Job drawing, mm, ordinate dimensions from the low corner. One solid piece. A direction names the side the tool comes from. Coordinates: 2 decimals unless noted, no trailing zeros. Write each loop counter-clockwise with the first axis right and the second up, starting at its lowest first coordinate (ties: lowest second). Pieces come first, ordered by that corner, then holes.
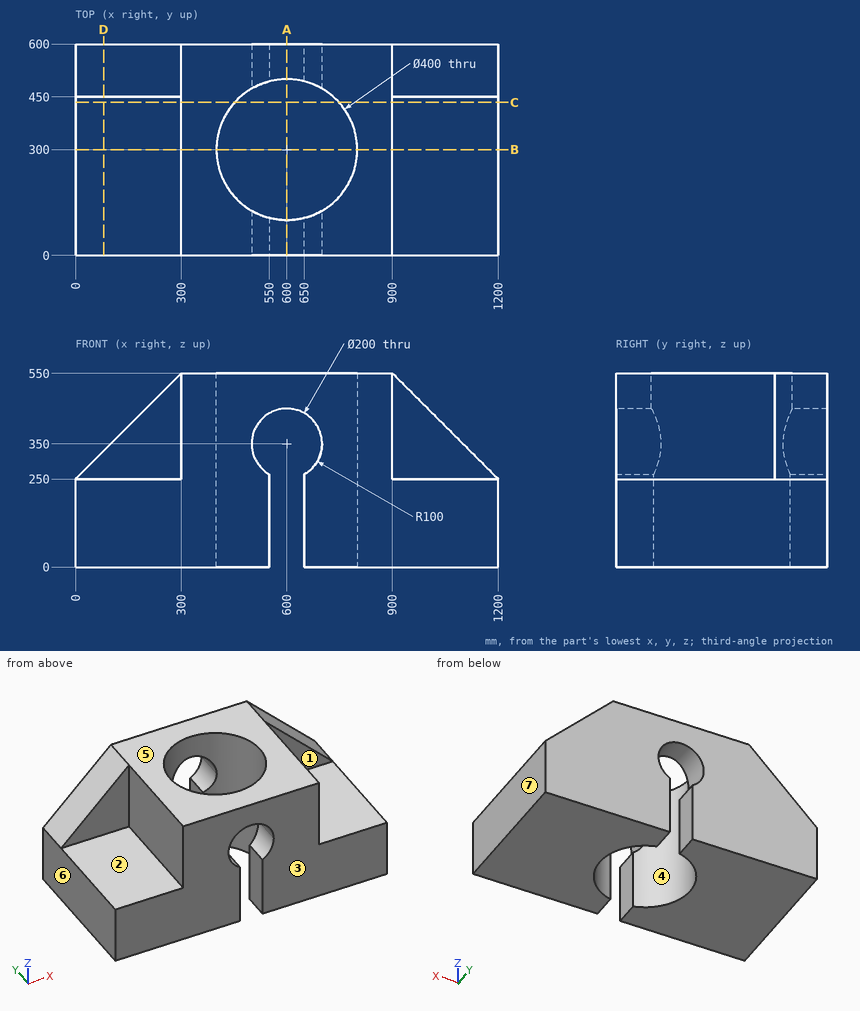
1. Saw through at B-B on y = 300. List the corners of the cut face in (x, z).
Computed values:
outline: (0, 0) - (400, 0) - (400, 550) - (300, 550) - (300, 250) - (0, 250) - close; (800, 0) - (1200, 0) - (1200, 250) - (900, 250) - (900, 550) - (800, 550) - close
2. Mould opens along X. For the marked faces 4, 5, 6 and 7 say: +X half, -X half, draft (parallel to the pull), parting line (faces both ways), or undercut.
Computed values:
face 4: undercut
face 5: draft
face 6: -X half
face 7: +X half
3. 3-axis set-ups, long thin cutter, end or side, ignore diameter. For the marked faces 1, 2 and 3: which of +Z, -Z, +X, -X, +Y, -Y reach the whole face in a straight line?
Computed values:
face 1: +Z, +X, -Y
face 2: +Z, -X, -Y
face 3: +Z, -Z, +X, -X, -Y
4. Saw through at A-A on x = 600. List the corners of the cut face in (y, z).
Computed values:
outline: (0, 450) - (100, 450) - (100, 550) - (0, 550) - close; (500, 450) - (600, 450) - (600, 550) - (500, 550) - close
5. Probe line 1 along X through (y, z) = (539, 39.5); line 2 along Z through (x, y) = (600, 53.5); line 3 along X through (y, z) = (167, 26.5). List the from-to ranges inside material, lowest first.
Computed values:
line 1: x = 0 to 550, 650 to 1200
line 2: z = 450 to 550
line 3: x = 0 to 450.63, 749.37 to 1200
6. Flat gauge pins, fed straight in: pin 1 (4 mm diameter, centred on y = 145, z = 342.5, fed in from +X); pin 2 (10 mm diameter, centred on y = 173.5, z = 156.5, fed in from -X); pin 3 (12 mm diameter, centred on y = 356, z = 396, fed in from -X). Where does each tip first touch, or does it go through?
Computed values:
pin 1: stops at x = 900
pin 2: stops at x = 0
pin 3: stops at x = 300
7. Saw through at D-D on x = 80. List the corners of the cut face in (y, z), plus the area to 3 significant figures.
Computed values:
outline: (0, 0) - (600, 0) - (600, 330) - (450, 330) - (450, 250) - (0, 250) - close
area: 162,000 mm2
8. Saw through at C-C on y = 434. List the corners of the cut face in (x, z), plus the area to 3 significant figures.
Computed values:
outline: (0, 0) - (451.53, 0) - (451.53, 550) - (300, 550) - (300, 250) - (0, 250) - close; (748.47, 0) - (1200, 0) - (1200, 250) - (900, 250) - (900, 550) - (748.47, 550) - close
area: 317,000 mm2
